Part model, mm, in its own coordinate system. Coordinates: 2 decimals unless noted, no trailing zeros. Write each loop counter-clockwise with the first axis right and the second up, starting at its lowest first coordinate (ties: lowest second). Pieces come first, ordered by that corner, then holes. Notation, with made-up numbers: (51, -29) - (72, -29) arc R12 ccw to (72, -21) - close; hole circle Ø7 at (-29, 61.5). An arc over 180 degrees is marked (long way). Use a Markdown table: item, result.
```python
from build123d import *

# Parameters (mm, degrees)
SKETCH1_R           = 2
SKETCH1_W           = 12.7
SKETCH1_H           = 50.8
BOSS_EXTRUDE3_DEPTH = 3.175


with BuildPart() as part:
    # Sketch1 → Boss-Extrude3 (new body)
    with BuildSketch(Plane(origin=(0, 0, 0), x_dir=(1, 0, 0), z_dir=(0, 1, 0))):
        with BuildLine():
            ThreePointArc((34.194833578, -66.63583839), (33.11372382, -66.748004461), (32.240681933, -66.10056535))
            ThreePointArc((32.240681933, -66.10056535), (0, -48.302004425), (-32.240681933, -66.10056535))
            ThreePointArc((-32.240681933, -66.10056535), (-33.11372382, -66.748004461), (-34.194833578, -66.63583839))
            ThreePointArc((-34.194833578, -66.63583839), (0, 74.897407173), (34.194833578, -66.63583839))
        make_face()
        with Locations((0, 53.061187965)):
            Circle(SKETCH1_R, mode=Mode.SUBTRACT)
        with Locations((18.178952795, 24.310551096)):
            Circle(SKETCH1_R, mode=Mode.SUBTRACT)
        with Locations((46.663733983, 40.081231883)):
            Circle(SKETCH1_R, mode=Mode.SUBTRACT)
        with Locations((46.663733983, -40.081231883)):
            Circle(SKETCH1_R, mode=Mode.SUBTRACT)
        with Locations((-46.663733983, -40.081231883)):
            Circle(SKETCH1_R, mode=Mode.SUBTRACT)
        with Locations((-18.178952795, 24.310551096)):
            Circle(SKETCH1_R, mode=Mode.SUBTRACT)
        with Locations((-46.663733983, 40.081231883)):
            Circle(SKETCH1_R, mode=Mode.SUBTRACT)
        with Locations((61.164123727, 0)):
            Rectangle(SKETCH1_W, SKETCH1_H, mode=Mode.SUBTRACT)
        with Locations((-61.164123727, 0)):
            Rectangle(SKETCH1_W, SKETCH1_H, mode=Mode.SUBTRACT)
        with BuildLine():
            ThreePointArc((-5.853899988, 60.78531778), (0.003726822, 57.376699875), (5.857575472, 60.791802193))
            ThreePointArc((5.857575472, 60.791802193), (10.16, 64.107698843), (5.857575472, 67.423595493))
            ThreePointArc((5.857575472, 67.423595493), (0.003726822, 70.838697812), (-5.853899988, 67.430079907))
            ThreePointArc((-5.853899988, 67.430079907), (-10.167207264, 64.107698843), (-5.853899988, 60.78531778))
        make_face(mode=Mode.SUBTRACT)
    extrude(amount=BOSS_EXTRUDE3_DEPTH)


solid = part.part
```
Item 1: Band-saw the part on B-B, the plane z = 0. Give the cut face in (x, y) (3 decimals), then the cut area to 3 significant figures.
From the geometry:
| item | result |
|---|---|
| outline | (-74.897, 0) - (-67.514, 0) - (-67.514, 3.175) - (-74.897, 3.175) - close; (-54.814, 0) - (54.814, 0) - (54.814, 3.175) - (-54.814, 3.175) - close; (67.514, 0) - (74.897, 0) - (74.897, 3.175) - (67.514, 3.175) - close |
| area | 395 mm^2 |
Item 2: Band-saw the part on D-D, the plane x = -62. Give the cut face in (y, z) (3 decimals), then the cut area to 3 significant figures.
From the geometry:
| item | result |
|---|---|
| outline | (0, -42.019) - (3.175, -42.019) - (3.175, -25.4) - (0, -25.4) - close; (0, 25.4) - (3.175, 25.4) - (3.175, 42.019) - (0, 42.019) - close |
| area | 106 mm^2 |
Item 3: Band-saw the part on C-C, the plane y = 1.7. Count the separate pieces of the cut face and the enclosed holes in it, then the cut area to 3 significant figures.
From the geometry:
| item | result |
|---|---|
| separate pieces | 1 |
| enclosed holes | 10 |
| area | 14,800 mm^2 |
Item 4: Drop flat-ended pins along their axis: P1, Ø1.6, axis at x = 60.5, y = 2.5, coming from the -Z side; P2, Ø1, axis at y = 2, z = -5, coming from the +X side; P3, Ø1, axis at x = 12.5, y = 1, coming from the -Z side; P4, Ø6.5, axis at x = 18.18, z = -24.31, coming from the +Y side (3 decimals). Give the stop position or say it passes through.
From the geometry:
| item | result |
|---|---|
| P1 | z = -45.23 |
| P2 | x = 74.76 |
| P3 | z = -73.93 |
| P4 | y = 3.175 |
Item 5: Two-plate mould, pull along Z, no slides. Class faces 1 (the face through (0.538, 1.565, 48.306)), 2 (the face through (-2.796, 1.565, -74.845)), 3 (the face through (-61, 2, 25.4)): pulls with the +Z half, pulls with the -Z half, needs draft (parallel to the pull), parting line crosses it, or undercut.
From the geometry:
| item | result |
|---|---|
| face 1 | pulls with the +Z half |
| face 2 | parting line crosses it |
| face 3 | undercut |
Item 6: Band-saw the part on A-A, the plane x = 0. Give the cut face in (y, z) (3 decimals), then the cut area to 3 significant figures.
From the geometry:
| item | result |
|---|---|
| outline | (0, -74.897) - (3.175, -74.897) - (3.175, -70.839) - (0, -70.839) - close; (0, -57.377) - (3.175, -57.377) - (3.175, -55.061) - (0, -55.061) - close; (0, -51.061) - (3.175, -51.061) - (3.175, 48.302) - (0, 48.302) - close |
| area | 336 mm^2 |
Item 7: Drill centre lines: probe 1 along X at (y, z) = (1.8, -13.5); probe 2 along Z at (x, y) = (0, 1.55); probe 3 along Z at (x, y) = (64.5, 2.7). Where is each one in solid material? Low to high.
From the geometry:
| item | result |
|---|---|
| probe 1 | -73.67 to -67.51, -54.81 to 54.81, 67.51 to 73.67 |
| probe 2 | -74.9 to -70.84, -57.38 to -55.06, -51.06 to 48.3 |
| probe 3 | -38.07 to -25.4, 25.4 to 38.07 |
